Here's how the part is built. I have some questions about the finished solid (model axes, mm). Face numbers are marked on the shaded views. Coordinates: 2 decimals unless noted, no trailing zeros. Loops run counter-clockwise (first coordinate to the right, second up) from the corner with the lowest first, then second, coordinate; pieces in that order, holes last. Notation, with made-up numbers: (74.25, 70.25) -> (103.25, 70.25) arc R17 cw to (103.25, 79.25) -> close; hole circle Ø4 at (-17.75, 24). An arc over 180 degrees is marked (long way). Answer as a JSON object with one key per item and string values. Group by question number.
Q1. I need wall thicknesses on line 1 (Y direction, x = 5, z = 2); line 2 (X direction, y = -0.15, z = 2.25); line 3 (Y direction, x = 4, z = 3.3). Which ranges of each line are inside material? Lowest first, please.
Q2. I want a section at C-C on z = 0.45. Write out the boundary of the cut face in (x, y).
Q3. Thinking about a two-plate mould opening in Y: for the marked faces 1, 2 and 3, which applies, released by +Y, released by -Y, zero draft, split by the parting line, or undercut?
Q4. I want a section at A-A on x = 5. Write out the boundary of the cut face in (y, z).
Q5. I'm going to push a flat-ended pin straight in: pin 1 (1.5 mm diameter, centred on y = -1, z = 0.5, fed in from +X). Where does the tip first touch, or does it pass through?
Q6. I want a section at B-B on y = 0. Write out the boundary of the cut face in (x, z).
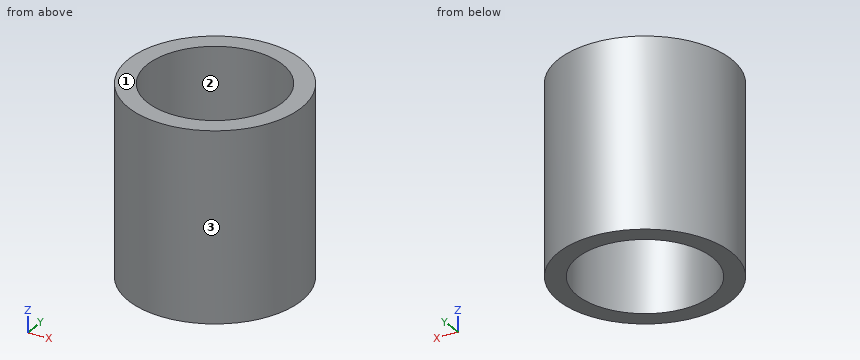
```python
from build123d import *

# Parameters (mm, degrees)
CYLINDER017_R     = 1.8
CYLINDER017_DEPTH = 5
CYLINDER016_R     = 2.3
CYLINDER016_DEPTH = 5


with BuildPart() as cylinder017:
    # Cylinder017 → Cylinder017 (new body)
    with BuildSketch(Plane(origin=(5, 0, -1), x_dir=(1, 0, 0), z_dir=(0, 0, 1))):
        Circle(CYLINDER017_R)
    extrude(amount=CYLINDER017_DEPTH)


with BuildPart() as cut007:
    # Cylinder016 → Cylinder016 (new body)
    with BuildSketch(Plane(origin=(5, 0, -1), x_dir=(1, 0, 0), z_dir=(0, 0, 1))):
        Circle(CYLINDER016_R)
    extrude(amount=CYLINDER016_DEPTH)

    # Cut007: cut Cylinder017
    add(cylinder017.part, mode=Mode.SUBTRACT)


solid = cut007.part
```
Result set:
{
 "1": {"line 1": "y = -2.3 to -1.8, 1.8 to 2.3", "line 2": "x = 2.7 to 3.21, 6.79 to 7.3", "line 3": "y = -2.07 to -1.5, 1.5 to 2.07"},
 "2": {"outline": "circle Ø4.6 at (5, 0); hole circle Ø3.6 at (5, 0)"},
 "3": {"face 1": "zero draft", "face 2": "undercut", "face 3": "split by the parting line"},
 "4": {"outline": "(-2.3, -1) -> (-1.8, -1) -> (-1.8, 4) -> (-2.3, 4) -> close; (1.8, -1) -> (2.3, -1) -> (2.3, 4) -> (1.8, 4) -> close"},
 "5": {"pin 1": "stops at x = 7.29"},
 "6": {"outline": "(2.7, -1) -> (3.2, -1) -> (3.2, 4) -> (2.7, 4) -> close; (6.8, -1) -> (7.3, -1) -> (7.3, 4) -> (6.8, 4) -> close"}
}
